from build123d import *


with BuildPart() as part:
    # Sketch1 → Base-Revolve (revolve)
    with BuildSketch(Plane.XY, mode=Mode.PRIVATE) as base_revolve_sk:
        with BuildLine():
            Line((50.8, 101.6), (50.8, 50.8))
            Line((50.8, 50.8), (76.2, 50.8))
            Line((76.2, 50.8), (101.6, 25.4))
            Line((101.6, 25.4), (101.6, 0))
            Line((101.6, 0), (127, 0))
            Line((127, 0), (127, 76.2))
            ThreePointArc((127, 76.2), (119.560512242, 94.160512242), (101.6, 101.6))
            Line((101.6, 101.6), (50.8, 101.6))
        make_face()
    revolve(base_revolve_sk.sketch.rotate(Axis((0, 127, 0), (0, -1, 0)), 90), axis=Axis((0, 127, 0), (0, -1, 0)))  # turned: the seam where the file's is


solid = part.part
Geometry check sheet. Reference: the model listing, model coordinates, mm. A direction names the side the tool comes from. Round coordinates to 2 decimals unless told otherwise and drop trailing zeros. Order: outer loops, then holes, each group sorted by start corner. A loop starts at its lowest first (then second) coordinate and runs counter-clockwise, first axis right, second up. Notation, with made-up numbers: M 56,66 L 86,66 A24 cw 86,78 Z; hole C -26,-25 d4. An arc over 180 degrees is marked long. Write each question's results on one line, items separated by ' | '. Start each with the question number.
1. Cross-section at C-C on y = 71. Record the boundary of the cut face in (x, z), plus the area to 3 significant figures.
2. Draft check along Z on faces 3 (the face through (123.98, 38.63, -27.53)), 4 (the face through (69.012, 49.211, 35.895)), 5 (the face through (-85, 0, 57)). Enter one of: pulls with the +Z half, pulls with the -Z half, needs draft (parallel to the pull), parting line crosses it, or undercut.
3. Material ranges on L1, parallel to X at y = 5, z = 0; L2, parallel to X at y = 73, z = 0; L3, parallel to Y at x = 23, z = -49.5, recorded low to high. Write a range as from..to.
4. Cross-section at B-B on x = 0. Record the boundary of the cut face in (y, z).
5. Cross-section at A-A on z = 0. Record the boundary of the cut face in (x, y), plus the area to 3 significant figures.
6. Set-up check for faces 1 (the face through (-47, 101.6, 21)), 2 (the face through (16, 50.8, -50)): record each of +Z, -Z, +X, -X, +Y, -Y from which the full face is reachable in a straight line by a thin tool's end or side.
7. Cross-section at D-D on y = 45.5. Record the boundary of the cut face in (x, z), plus the area to 3 significant figures.
8. Go/stop test with flat-tipped pins: P1, Ø2, axis at y = 90, z = 47.5, coming from the -X side; P2, Ø2, axis at x = 62.5, z = 47, coming from the -Y side; P3, Ø4, axis at x = -92, y = 14, coming from the -Z side. Record where each tip stops, or that it passes through.
Resolved:
1) outline: C 0,0 d254; hole C 0,0 d101.6 | area: 42,600 mm2
2) face 3: parting line crosses it | face 4: undercut | face 5: needs draft
3) L1: -127..-101.6, 101.6..127 | L2: -127..-50.8, 50.8..127 | L3: 50.8..101.6
4) outline: M 0,-127 L 76.2,-127 A25.4 ccw 101.6,-101.6 L 101.6,-50.8 L 50.8,-50.8 L 50.8,-76.2 L 25.4,-101.6 L 0,-101.6 Z; M 0,101.6 L 25.4,101.6 L 50.8,76.2 L 50.8,50.8 L 101.6,50.8 L 101.6,101.6 A25.4 ccw 76.2,127 L 0,127 Z
5) outline: M -127,0 L -101.6,0 L -101.6,25.4 L -76.2,50.8 L -50.8,50.8 L -50.8,101.6 L -101.6,101.6 A25.4 ccw -127,76.2 Z; M 50.8,50.8 L 76.2,50.8 L 101.6,25.4 L 101.6,0 L 127,0 L 127,76.2 A25.4 ccw 101.6,101.6 L 50.8,101.6 Z | area: 10,700 mm2
6) face 1: +Z, -Z, +X, -X, +Y | face 2: -Y
7) outline: C 0,0 d254; hole C 0,0 d163 | area: 29,800 mm2
8) P1: x = -114.16 | P2: y = 47.8 | P3: z = -89.6
